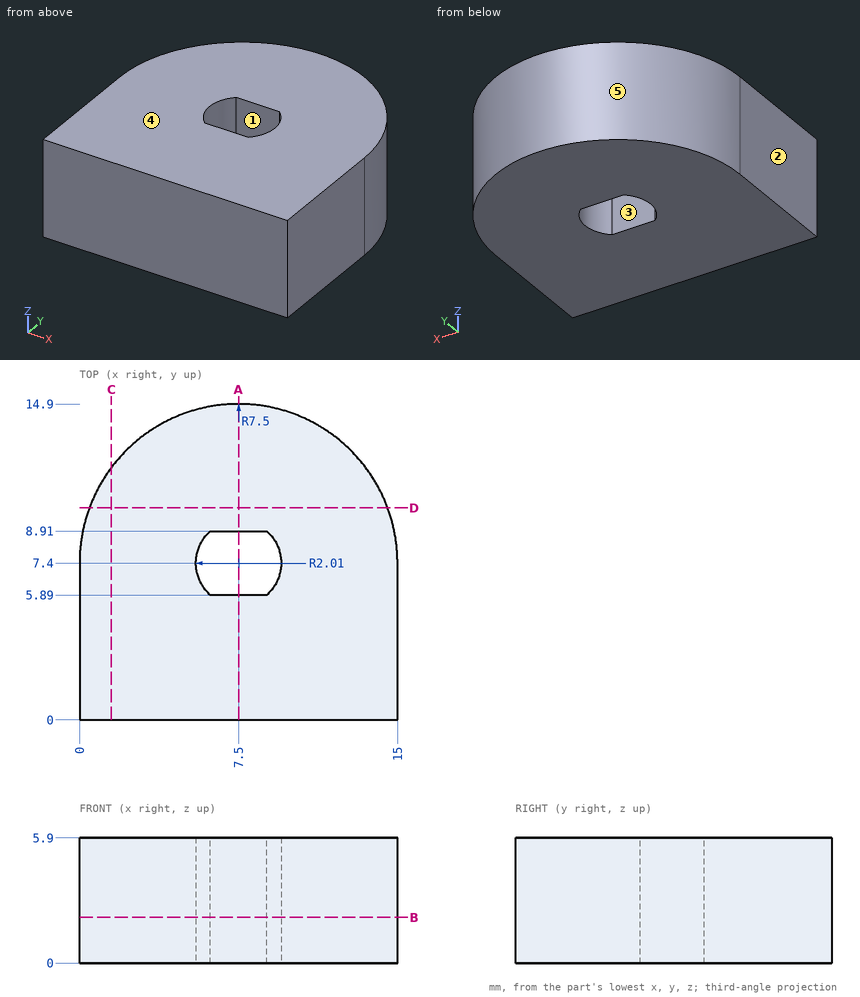
Could you check a few things on this drawing? It's one solid part, dimensions in mm from its lowest x, y, z. A direction names the side the tool comes from. Coordinates: 2 decimals unless noted, no trailing zeros. Write each loop counter-clockwise with the first axis right and the second up, starting at its lowest first coordinate (ties: lowest second). Pieces come first, ordered by that corner, then holes.
1) I'm going to push flat-ended pins straight in: pin 1 (1 mm diameter, centred on y = 10.5, z = 2.5, fed in from +X); pin 2 (2 mm diameter, centred on x = 3.5, z = 1.5, fed in from +Y). Where does each tip first touch, or does it pass through?
Filled in:
pin 1: stops at x = 14.53
pin 2: stops at y = 14.27
2) If we section it at A-A (x = 7.5): List the corners of the cut face in (y, z) for me.
Filled in:
outline: (0, 0) - (5.89, 0) - (5.89, 5.9) - (0, 5.9) - close; (8.91, 0) - (14.9, 0) - (14.9, 5.9) - (8.91, 5.9) - close
3) If we section it at D-D (y = 10): List the corners of the cut face in (x, z) for me.
Filled in:
outline: (0.47, 0) - (14.53, 0) - (14.53, 5.9) - (0.47, 5.9) - close
4) If we section it at B-B (z = 2.15): List the corners of the cut face in (x, y) for me, plus the area to 3 significant figures.
Filled in:
outline: (0, 0) - (15, 0) - (15, 7.4) arc R7.5 ccw to (0, 7.4) - close; hole (6.17, 5.89) - (8.83, 5.89) arc R2.01 ccw to (8.83, 8.91) - (6.17, 8.91) arc R2.01 ccw to start
area: 188 mm2
5) If I drill on line 1 (Y direction, x = 8.25, z = 1.05); line 2 (Y direction, x = 9.25, z = 3.7); line 3 (X direction, y = 7.75, z = 4.5), over which ranges is the centre line in solid material (lowest first)?
Filled in:
line 1: y = 0 to 5.89, 8.91 to 14.86
line 2: y = 0 to 6.41, 8.39 to 14.69
line 3: x = 0.01 to 5.52, 9.48 to 14.99
6) Thinking about a two-plate mould opening in X: for the marked faces 3, 4 and 5, which applies, +X half, -X half, draft (parallel to the pull), parting line (faces both ways), or undercut?
Filled in:
face 3: undercut
face 4: draft
face 5: parting line
7) Which directions (+Z, -Z, +X, -X, +Y, -Y) give clear straight access to the entire face, cutting with the end or side of a thin tool? Please do the marked faces 1 and 2.
Filled in:
face 1: +Z, -Z
face 2: +Z, -Z, -X, +Y, -Y
8) If we section it at C-C (x = 1.5): List the corners of the cut face in (y, z) for me, plus the area to 3 significant figures.
Filled in:
outline: (0, 0) - (11.9, 0) - (11.9, 5.9) - (0, 5.9) - close
area: 70.2 mm2
